Design review of the part built by this model. Coordinates are the model's own, in mm. Give positions to 0.01 mm unless a question says otherwise; leave off trailing zeros. Order: outer loops, then holes, each group sorted by start corner. A loop starts at its lowest first (then second) coordinate and runs counter-clockwise, first axis right, second up. Notation, with made-up numbers: (20.25, -1.75) -> (37.25, -1.75) arc R23 cw to (37.25, 15.25) -> close; hole circle Ø2 at (-32, 7.5). An arc over 180 degrees is marked (long way). One line per item, written item: value. Start each with the question number.
1) Consider section A-A (y = -1.9). State the section outline as (x, z) points.
2) Consider section C-C (x = 247.5). State the section outline as (y, z) points.
3) Wall thickness on line 1 along X through (y, z) = (-4.7, 36); line 2 along Z through (x, y) = (293.5, -4.55); line 3 along Z through (x, y) = (36.5, -3.75): over which ranges is each line inside the solid? List them lowest first. Write a range as from..to.
4) Consider section B-B (z = 44). State the section outline as (x, y) points, plus the area to 4 significant figures.
5) For pin 1 (2 mm diameter, centred on x = 69.5, z = 18, fed in from +Y); pin 2 (2.5 mm diameter, centred on x = 85.5, y = -3, fed in from +Z), all flat-tipped, find the tip position at first contact; note any pin that passes through.
from build123d import *

# Parameters (mm, degrees)
F1_DEPTH = 5


with BuildPart() as f1:
    # F0 (on Front) → F1 (new body)
    with BuildSketch(Plane.XZ):
        with BuildLine():
            Line((0, 35), (0, 0))
            Line((0, 0), (180, 0))
            Line((180, 0), (360, 0))
            Line((360, 0), (360, 35))
            ThreePointArc((360, 35), (358.535534, 38.535534), (355, 40))
            Line((355, 40), (320, 40))
            ThreePointArc((320, 40), (317.401719, 39.656549), (314.981915, 38.649788))
            Line((314.981915, 38.649788), (311.018085, 36.350212))
            ThreePointArc((311.018085, 36.350212), (308.598281, 35.343451), (306, 35))
            Line((306, 35), (240, 35))
            ThreePointArc((240, 35), (235.527864, 36.055728), (232, 39))
            Line((232, 39), (223, 51))
            ThreePointArc((223, 51), (219.472136, 53.944272), (215, 55))
            Line((215, 55), (180, 55))
            Line((180, 55), (145, 55))
            ThreePointArc((145, 55), (140.527864, 53.944272), (137, 51))
            Line((137, 51), (128, 39))
            ThreePointArc((128, 39), (124.472136, 36.055728), (120, 35))
            Line((120, 35), (54, 35))
            ThreePointArc((54, 35), (51.401719, 35.343451), (48.981915, 36.350212))
            Line((48.981915, 36.350212), (45.018085, 38.649788))
            ThreePointArc((45.018085, 38.649788), (42.598281, 39.656549), (40, 40))
            Line((40, 40), (5, 40))
            ThreePointArc((5, 40), (1.464466, 38.535534), (0, 35))
        make_face()
    extrude(amount=F1_DEPTH)


solid = f1.part
Checked values:
1. outline: (0, 0) -> (360, 0) -> (360, 35) arc R5 ccw to (355, 40) -> (320, 40) arc R10 ccw to (314.98, 38.65) -> (311.02, 36.35) arc R10 cw to (306, 35) -> (240, 35) arc R10 cw to (232, 39) -> (223, 51) arc R10 ccw to (215, 55) -> (145, 55) arc R10 ccw to (137, 51) -> (128, 39) arc R10 cw to (120, 35) -> (54, 35) arc R10 cw to (48.98, 36.35) -> (45.02, 38.65) arc R10 ccw to (40, 40) -> (5, 40) arc R5 ccw to (0, 35) -> close
2. outline: (-5, 0) -> (0, 0) -> (0, 35) -> (-5, 35) -> close
3. line 1: x = 0.1..49.64, 124.36..235.64, 310.36..359.9
3. line 2: z = 0..35
3. line 3: z = 0..40
4. outline: (131.75, -5) -> (228.25, -5) -> (228.25, 0) -> (131.75, 0) -> close
4. area: 482.5 mm^2
5. pin 1: stops at y = 0
5. pin 2: stops at z = 35
